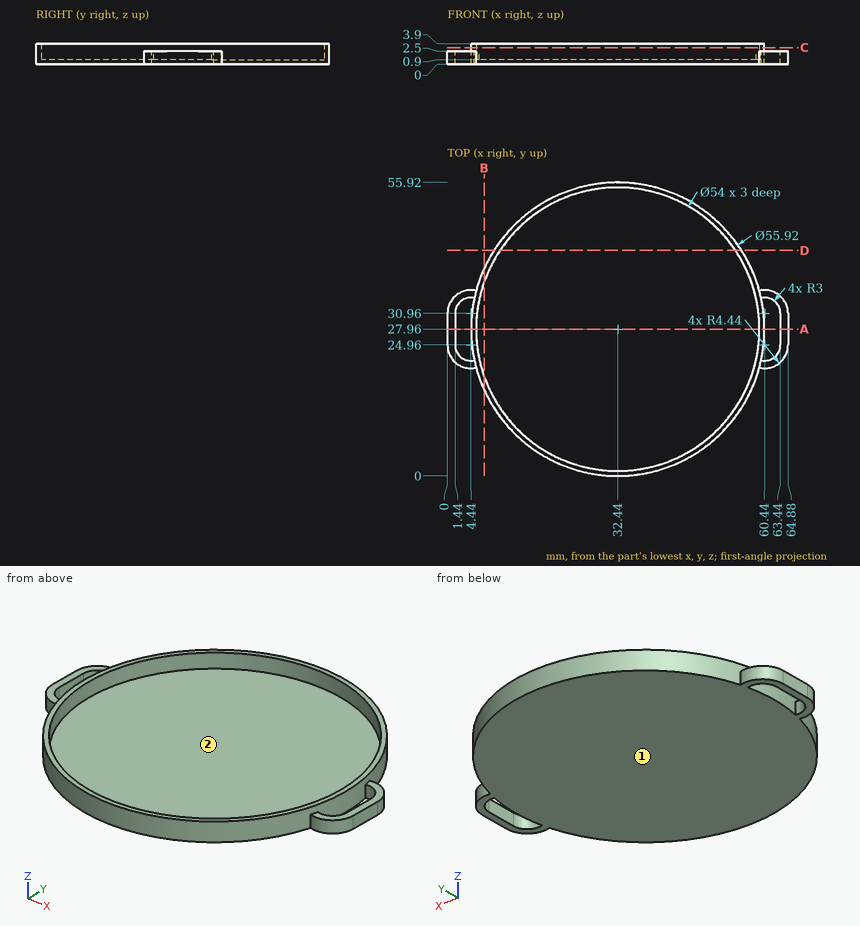
Input: dimensioned drawing with shaded views. Units: mm. Origin: part minimum x, y, z. Round coordinates to 2 decimals unless told otherwise and drop trailing zeros. Order: outer loops, then holes, each group sorted by start corner. A loop starts at its lowest first (then second) coordinate and runs counter-clockwise, first axis right, second up. Notation, with made-up numbers: (26.5, -36.75) - (57.5, -36.75) arc R21 ccw to (57.5, -17.75) - close; hole circle Ø4 at (-37.75, -4). An arc over 180 degrees is marked (long way). Write item = value, one per line. Start each with the question number.
Q1. Cut plane B-B on x = 7. Return the cut outline in (y, z).
Q2. Cut plane D-D on y = 43. Return the cut outline in (x, z).
Q3. Cut plane C-C on z = 3.2. Return the cut outline in (x, y), and give its area (3 significant figures).
Q4. Cut plane A-A on y = 27.96. Return the cut outline in (x, z), and give its area (3 significant figures).
Q5. Pin query (flat end, axial travel): pin 1 (4 mm diameter, centred on x = 33, y = 26.5, fed in from +Z); pin 2 (6 mm diameter, centred on x = 62, y = 28, fed in from +Z); pin 3 (1.6 mm diameter, centred on x = 1.5, y = 26, fed in from +Z); pin 4 (1.5 mm diameter, centred on y = 38.5, z = 0.5, fed in from -X). Return the tip coordinate at first contact, or that it passes through.
Q6. Ray query, line 1 (X direction, y = 27.96, z = 2.05); line 2 (Y direction, x = 32.44, z = 2.35); line 3 (X direction, y = 27.96, z = 2.9). Return the intervals inside material, ascending. Write a range as from..to.
Q7. Pull-direction query (X, two-part tool) for the marked faces 1 and 2; classes: +X half, -X half, draft (parallel to the pull), parting line (faces both ways), or undercut.
Outcome:
q1.outline = (16.36, 0) - (39.56, 0) - (39.56, 3.9) - (37, 3.9) - (37, 0.9) - (18.92, 0.9) - (18.92, 3.9) - (16.36, 3.9) - close
q2.outline = (8.87, 0) - (56.01, 0) - (56.01, 3.9) - (54.86, 3.9) - (54.86, 0.9) - (10.02, 0.9) - (10.02, 3.9) - (8.87, 3.9) - close
q3.outline = circle Ø55.92 at (32.44, 27.96); hole circle Ø54 at (32.44, 27.96)
q3.area = 166 mm^2
q4.outline = (0, 0) - (1.44, 0) - (1.44, 2.5) - (0, 2.5) - close; (4.48, 0) - (60.4, 0) - (60.4, 3.9) - (59.44, 3.9) - (59.44, 0.9) - (5.44, 0.9) - (5.44, 3.9) - (4.48, 3.9) - close; (63.44, 0) - (64.88, 0) - (64.88, 2.5) - (63.44, 2.5) - close
q4.area = 63.3 mm^2
q5.pin_1 = 0.9
q5.pin_2 = 3.9
q5.pin_3 = 2.5
q5.pin_4 = 6.25
q6.line_1 = 0..1.44, 4.48..5.44, 59.44..60.4, 63.44..64.88
q6.line_2 = 0..0.96, 54.96..55.92
q6.line_3 = 4.48..5.44, 59.44..60.4
q7.face_1 = draft
q7.face_2 = undercut
